Job drawing, mm, ordinate dimensions from the low corner. One solid piece. Give positions to 0.01 mm unless a question says otherwise; leave off trailing zeros. Write each loop counter-clockwise with the first axis right and the second up, starting at its lowest first coordinate (ties: lowest second). Pieces come first, ordered by that corner, then holes. Notation, with made-up numbers: M 3,-22.5 L 45,-22.5 A22 ccw 45,-7.5 Z; hole C 61.5,46.5 d9. An arc over 180 degrees is marked long. Use a Markdown table: item, result.
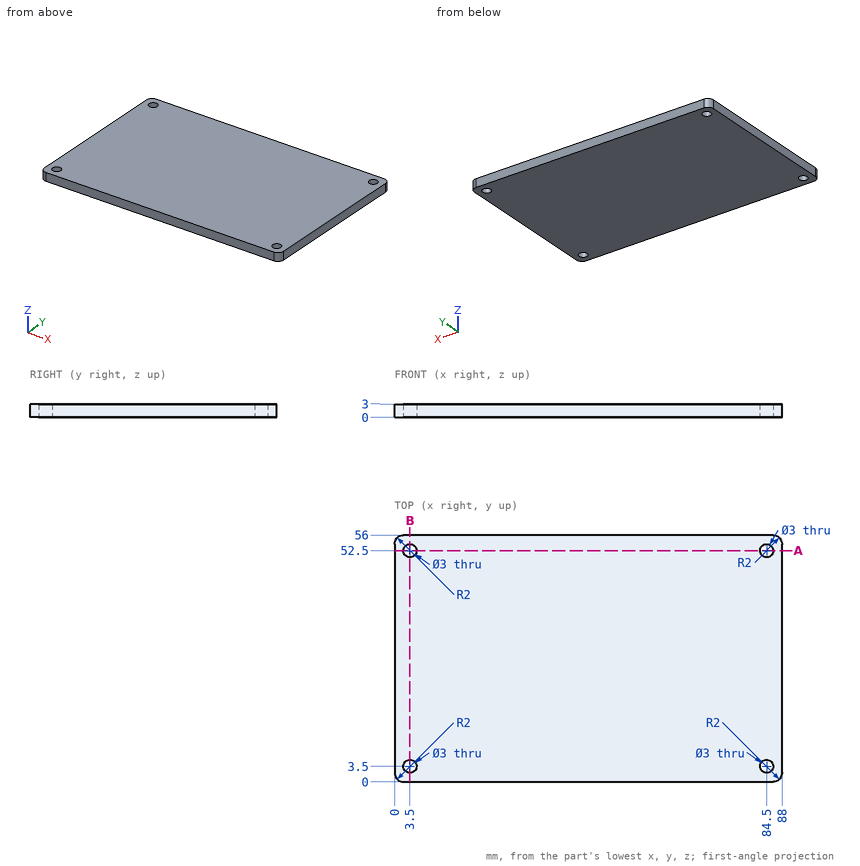
1. Cut at A-A, the plane y = 52.5. Give the cut face in (x, z), then the cut area to 3 significant figures.
Findings below:
| item | result |
|---|---|
| outline | M 0,0 L 2,0 L 2,3 L 0,3 Z; M 5,0 L 83,0 L 83,3 L 5,3 Z; M 86,0 L 88,0 L 88,3 L 86,3 Z |
| area | 246 mm2 |
2. Drill centre lines: L1, parallel to Y at x = 84.5, z = 2.1; L2, parallel to X at y = 3.5, z = 2.1. Where is each one in solid material? Low to high.
Findings below:
| item | result |
|---|---|
| L1 | 0 to 2, 5 to 51, 54 to 56 |
| L2 | 0 to 2, 5 to 83, 86 to 88 |
3. Cut at B-B, the plane x = 3.5. Give the cut face in (y, z).
Findings below:
| item | result |
|---|---|
| outline | M 0,0 L 2,0 L 2,3 L 0,3 Z; M 5,0 L 51,0 L 51,3 L 5,3 Z; M 54,0 L 56,0 L 56,3 L 54,3 Z |
